from build123d import *

# Parameters (mm, degrees)
BOSS_EXTRUDE1_DEPTH  = 4.2
FILLET2_R            = 3
FILLET5_R            = 3
SKETCH3_R            = 2.1
CUT_EXTRUDE1_DEPTH   = 16
FILLET6_R            = 3
FILLET2_OF_MIRROR1_R = 3
FILLET5_OF_MIRROR1_R = 3
FILLET6_OF_MIRROR1_R = 3


with BuildPart() as part:
    # Sketch2 → Boss-Extrude1 (new body, symmetric)
    with BuildSketch(Plane(origin=(0, 0, 0), x_dir=(1, 0, 0), z_dir=(0, 1, 0))):
        with BuildLine():
            Line((0, 0), (-24, 0))
            ThreePointArc((-24, 0), (-50.506230897, -3.686965816), (-75, -14.467933694))
            Line((-75, -14.467933694), (-77.100442165, -11.063797576))
            ThreePointArc((-77.100442165, -11.063797576), (-52.558629139, -0.11650046), (-26, 3.980220055))
            Line((-26, 3.980220055), (-26, 8))
            Line((-26, 8), (-29.5, 8))
            Line((-29.5, 8), (-29.5, 23))
            Line((-29.5, 23), (-27.5, 23))
            Line((-27.5, 23), (-27.5, 10))
            Line((-27.5, 10), (-24, 10))
            Line((-24, 10), (-20.5, 10))
            Line((-20.5, 10), (-20.5, 23))
            Line((-20.5, 23), (-18.5, 23))
            Line((-18.5, 23), (-18.5, 8))
            Line((-18.5, 8), (-22, 8))
            Line((-22, 8), (-22, 4))
            Line((-22, 4), (0, 4))
            Line((0, 4), (0, 0))
        make_face()
    boss_extrude1 = extrude(amount=BOSS_EXTRUDE1_DEPTH, both=True)

    # Fillet2
    fillet2_edges = [part.edges().sort_by_distance(p)[0] for p in [
        (-29.5, 0, -8),
    ]]
    fillet(fillet2_edges, radius=FILLET2_R)

    # Fillet5
    fillet5_edges = [part.edges().sort_by_distance(p)[0] for p in [
        (-26, 0, -3.980220055),
        (-18.5, 0, -8),
        (-22, 0, -4),
    ]]
    fillet(fillet5_edges, radius=FILLET5_R)

    # Sketch3 → Cut-Extrude1 (cut)
    with BuildSketch(Plane(origin=(-18.5, 0, 0), x_dir=(0, 0, -1), z_dir=(1, 0, 0))):
        with Locations((20, 0)):
            Circle(SKETCH3_R)
    cut_extrude1 = extrude(amount=-CUT_EXTRUDE1_DEPTH, mode=Mode.SUBTRACT)

    # Fillet6
    fillet6_edges = [part.edges().sort_by_distance(p)[0] for p in [
        (-27.5, 0, -10),
        (-20.5, 0, -10),
    ]]
    fillet(fillet6_edges, radius=FILLET6_R)

    # Mirror1: Boss-Extrude1, Cut-Extrude1 across plane
    add(boss_extrude1.mirror(Plane(origin=(0, -4.2, -4), x_dir=(0, 0, 1), z_dir=(1, 0, 0))))
    add(cut_extrude1.mirror(Plane(origin=(0, -4.2, -4), x_dir=(0, 0, 1), z_dir=(1, 0, 0))), mode=Mode.SUBTRACT)

    # Fillet2 of Mirror1
    fillet2_of_mirror1_edges = [part.edges().sort_by_distance(p)[0] for p in [
        (29.5, 0, -8),
    ]]
    fillet(fillet2_of_mirror1_edges, radius=FILLET2_OF_MIRROR1_R)

    # Fillet5 of Mirror1
    fillet5_of_mirror1_edges = [part.edges().sort_by_distance(p)[0] for p in [
        (26, 0, -3.980220055),
        (18.5, 0, -8),
        (22, 0, -4),
    ]]
    fillet(fillet5_of_mirror1_edges, radius=FILLET5_OF_MIRROR1_R)

    # Fillet6 of Mirror1
    fillet6_of_mirror1_edges = [part.edges().sort_by_distance(p)[0] for p in [
        (27.5, 0, -10),
        (20.5, 0, -10),
    ]]
    fillet(fillet6_of_mirror1_edges, radius=FILLET6_OF_MIRROR1_R)


solid = part.part
Geometry: final body of the model. Coordinates: model frame, mm. A direction names the side the tool comes from. Give positions to 0.01 mm unless a question says otherwise; leave off trailing zeros. Loops run counter-clockwise (first coordinate to the right, second up) from the corner with the lowest first, then second, coordinate; pieces in that order, holes last. Notation, with made-up numbers: M 44,63 L 60,63 A15 ccw 60,74 Z; hole C -9,8 d5. An arc over 180 degrees is marked long. Put each result on its own line as item: value.
1) Reachability of faces 1 (the cylindrical face through (26.64, -0.06, -10.9)), 2 (the cylindrical face through (-50.144, 0.059, 3.585)), 3 (the cylindrical face through (-28.64, -0.06, -8.9)), 4 (the cylindrical face through (-21.1, 0.06, -4.86)), 5 (the cylindrical face through (28.6, -0.06, -8.86)) from +Z, -Z, +X, -X, +Y, -Y: full face, straight path, thin tool, end or side. Return the list, or none.
Computed values:
face 1: -Z, +Y, -Y
face 2: +Z, +Y, -Y
face 3: -X, +Y, -Y
face 4: +Y, -Y
face 5: +X, +Y, -Y
2) First-contact query: P1, Ø3.5, axis at y = 0, z = -20, coming from the +X side; P2, Ø5, axis at y = 0, z = -20, coming from the -X side; P3, Ø2, axis at x = -44.5, y = 2, coming from the +Z side; P4, Ø0.9, axis at y = 0.5, z = -7.5, coming from the +X side. Flat tips, straight axial feed; report the tip coordinate or a pass-through.
Computed values:
P1: passes through
P2: stops at x = -29.5
P3: stops at z = 2.41
P4: stops at x = 26
3) Cut plane D-D, the plane x = 0. Return the cut outline in (y, z), plus the area to 3 significant figures.
Computed values:
outline: M -4.2,-4 L 4.2,-4 L 4.2,0 L -4.2,0 Z
area: 33.6 mm^2
4) Cut plane C-C, the plane z = 9. Return the cut outline in (x, y), plus the area to 3 significant figures.
Computed values:
outline: M -73.6,-4.2 L -64.83,-4.2 L -64.83,4.2 L -73.6,4.2 Z; M 64.83,-4.2 L 73.6,-4.2 L 73.6,4.2 L 64.83,4.2 Z
area: 147 mm^2
5) Cut plane A-A, the plane z = -20. Give the number of separate pieces and of enclosed holes in the cut face, plus the area to 3 significant figures.
Computed values:
separate pieces: 8
enclosed holes: 0
area: 33.6 mm^2
6) Mould query, pull axis Y, two halves, no side actions, for faces 6 (the cylindrical face through (19.486, 0.631, -22.003)), 7 (the cylindrical face through (50.144, 0.059, 3.585)), 8 (the flat face through (0, 4.2, -2)), 9 (the cylindrical face through (28.486, 0.631, -22.003)). Classes: released by +Y, released by -Y, zero draft, split by the parting line, or undercut.
Computed values:
face 6: undercut
face 7: zero draft
face 8: released by +Y
face 9: undercut
7) Material intervals for L1, parallel to X at y = -3, z = -19.5; L2, parallel to Y at x = -19, z = -20; L3, parallel to X at y = -1.5, z = -11.5, sorted ascending. Write a range as from..to.
Computed values:
L1: x = -29.5..-27.5, -20.5..-18.5, 18.5..20.5, 27.5..29.5
L2: y = -4.2..-2.1, 2.1..4.2
L3: x = -29.5..-27.1, -20.9..-18.5, 18.5..20.9, 27.1..29.5
